Read the model definition and answer for the solid it produces. Units are mm, in the model's axes. Coordinates: 2 decimals unless noted, no trailing zeros. Loops run counter-clockwise (first coordinate to the right, second up) from the corner with the lowest first, then second, coordinate; pieces in that order, holes last. Notation, with made-up numbers: (29, -2.5) -> (88, -2.5) arc R9 ccw to (88, 14.5) -> close; hole circle Ø10 at (75.5, 44). An arc over 180 degrees is marked (long way). Answer as a JSON object with one key per item and string values. Group by question number.
Q1. Straight lines are drawn through the part: line 1 along Y through (x, z) = (0, 1.2) (3 decimals); line 2 along Y through (x, z) = (-0.55, 1.3); line 3 along Y through (x, z) = (-1.1, 0.5). For each, find the intervals that lie inside material, in ascending order. Write a range as [from, to].
Q2. Determine the mould class of faces 1 (the cylindrical face through (-0.08, 18.16, 0.99)), 2 (the flat face through (-1.25, 10, 1)), 3 (the cylindrical face through (-0.03, 20.03, 0.99)) for opening direction X: released by +X, released by -X, zero draft, split by the parting line, or undercut.
Q3. The part is cut by section B-B on z = 1.35. Write down the section's boundary in (x, y) (3 decimals).
Q4. The part is cut by section A-A on x = 0. Write down the section's boundary in (y, z) (3 decimals).
Q5. The part is cut by section C-C on x = -1.05. Write down the section's boundary in (y, z).
Q6. This flat-tipped pin is pushed along its axis until it touches: P1, Ø1, axis at x = 0, y = 18.78, coming from the -Z side. Where does it stop, or does it pass through?
Autodesk Inventor part; units mm, degrees
ref_plane "YZ Plane" through (0, 0, 0) normal (1, 0, 0) x (0, 1, 0)
ref_plane "XZ Plane" through (0, 0, 0) normal (0, 1, 0) x (-1, 0, 0)
ref_plane "XY Plane" through (0, 0, 0) normal (0, 0, 1) x (1, 0, 0)
sketch "草圖1" plane through (0, 0, 0) normal (0, 0, 1) x (1, 0, 0)
  line L0 (0, 0) -> (0, 18.78) construction
  line L1 (1.25, 0) -> (1.25, 18.78)
  line L2 (-1.25, 18.78) -> (-1.25, 0)
  arc A0 (-1.25, 0) -> (1.25, 0) centre (0, 0) ccw
  arc A1 (1.25, 18.78) -> (-1.25, 18.78) centre (0, 18.78) ccw
  circle A2 centre (0, 18.78) radius 0.625
  circle A3 centre (0, 0) radius 0.625
  point P0 (0, 9.39)
  dimension "d0" = 18.78
  dimension "d1" = 2.5
  dimension "d2" = 1.25
  dimension "d3" = 1.25
extrude "擠出1" add sketch "草圖1" along normal blind 2
properties part number "1"
Final values:
{
 "1": {"line 1": "y = [-1.25, -0.625], [0.625, 18.155], [19.405, 20.03]", "line 2": "y = [-1.12, -0.3], [0.3, 18.48], [19.08, 19.9]", "line 3": "y = [-0.59, 19.37]"},
 "2": {"face 1": "undercut", "face 2": "released by -X", "face 3": "split by the parting line"},
 "3": {"outline": "(-1.25, 0) arc R1.25 ccw to (1.25, 0) -> (1.25, 18.78) arc R1.25 ccw to (-1.25, 18.78) -> close; hole circle Ø1.25 at (0, 0); hole circle Ø1.25 at (0, 18.78)"},
 "4": {"outline": "(-1.25, 0) -> (-0.625, 0) -> (-0.625, 2) -> (-1.25, 2) -> close; (0.625, 0) -> (18.155, 0) -> (18.155, 2) -> (0.625, 2) -> close; (19.405, 0) -> (20.03, 0) -> (20.03, 2) -> (19.405, 2) -> close"},
 "5": {"outline": "(-0.68, 0) -> (19.46, 0) -> (19.46, 2) -> (-0.68, 2) -> close"},
 "6": {"P1": "passes through"}
}
